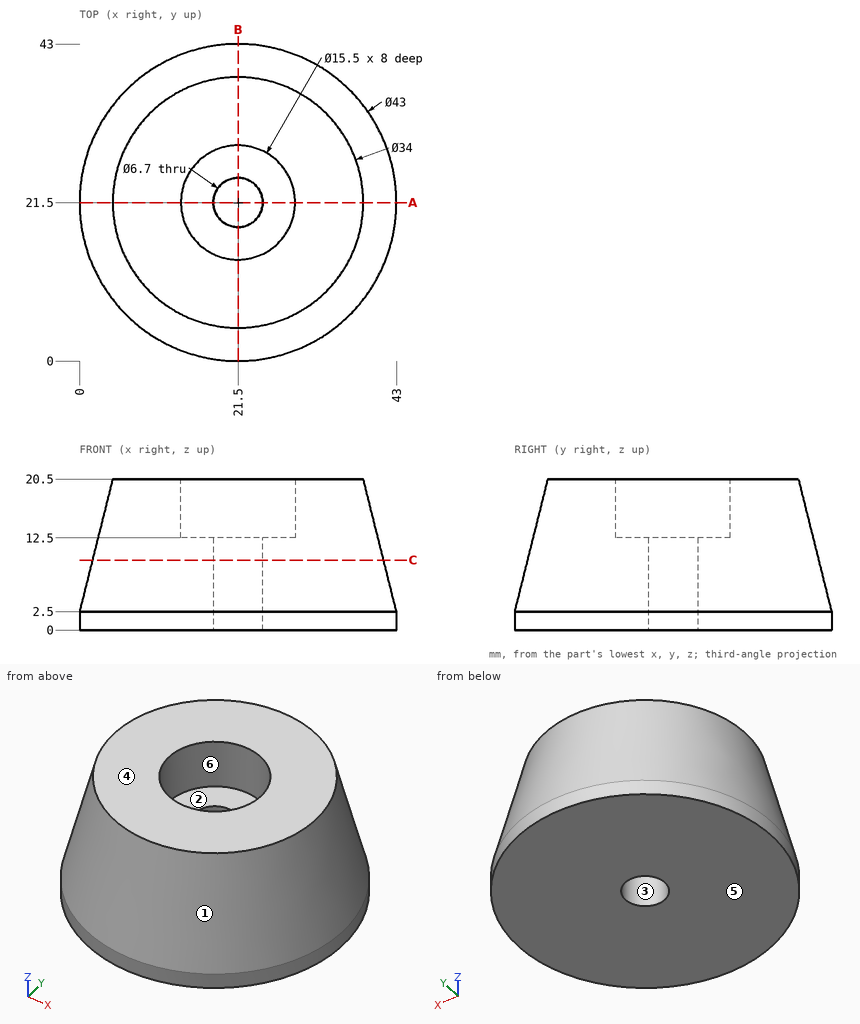
Part print with two shaded views. Sizes in mm from the minimum x, y, z corner. A direction names the side the tool comes from. Round coordinates to 2 decimals unless told otherwise and drop trailing zeros. Loops run counter-clockwise (first coordinate to the right, second up) from the corner with the lowest first, then second, coordinate; pieces in that order, holes last. Notation, with made-up numbers: M 13.25,-3 L 70.25,-3 A8 cw 70.25,6 Z; hole C -22.75,9.5 d2. An arc over 180 degrees is marked long. Put each result on its own line as item: value. Start each with the question number.
Item 1: 3-axis set-ups, long thin cutter, end or side, ignore diameter. For the marked faces 5 and 6: which of +Z, -Z, +X, -X, +Y, -Y reach the whole face in a straight line?
Item 2: Cut at A-A (y = 21.5). List the corners of the cut face in (x, z).
Item 3: Mould opens along Y. For the marked faces 1, 2, 3 and 4 say: released by +Y, released by -Y, zero draft, split by the parting line, or undercut.
Item 4: Drill centre lines: line 1 along Y through (x, z) = (24, 9.25); line 2 along Z through (x, y) = (17, 22.5); line 3 along Y through (x, z) = (21.5, 2.75). Where is each one in solid material? Low to high.
Item 5: Cut at C-C (z = 9.5). List the corners of the cut face in (x, y), then the cut area to 3 significant figures.
Item 6: Drop flat-ended pins along their axis: P1, Ø2, axis at x = 21.5, z = 16.5, coming from the -Y side; P2, Ø12.5, axis at x = 21.5, y = 21.5, coming from the +Z side; P3, Ø6, axis at x = 6, z = 11.5, coming from the +Y side. Give the stop position or say it passes through.
Answer block:
1. face 5: -Z, +X, -X, +Y, -Y
1. face 6: +Z
2. outline: M 0,0 L 18.15,0 L 18.15,12.5 L 13.75,12.5 L 13.75,20.5 L 4.5,20.5 L 0,2.5 Z; M 24.85,0 L 43,0 L 43,2.5 L 38.5,20.5 L 29.25,20.5 L 29.25,12.5 L 24.85,12.5 Z
3. face 1: split by the parting line
3. face 2: undercut
3. face 3: undercut
3. face 4: zero draft
4. line 1: 1.85 to 19.27, 23.73 to 41.15
4. line 2: 0 to 12.5
4. line 3: 0.06 to 18.15, 24.85 to 42.94
5. outline: C 21.5,21.5 d39.5; hole C 21.5,21.5 d6.7
5. area: 1,190 mm2
6. P1: y = 3.25
6. P2: z = 12.5
6. P3: y = 36.32
